Can you work these out from the drawing? Everything is in mm from the part's minimum corner. A direction names the side the tool comes from. Coordinates: 2 decimals unless noted, no trailing zeros. Order: outer loops, then holes, each group sorted by start corner. A loop starts at its lowest first (then second) coordinate and runs counter-clockwise, first axis right, second up. Notation, with made-up numbers: (19, 48) -> (62, 48) arc R15 ccw to (62, 61) -> close; hole circle Ø8 at (43.5, 42.5). An arc over 180 degrees is marked (long way). Answer in a Markdown table with one row per item.
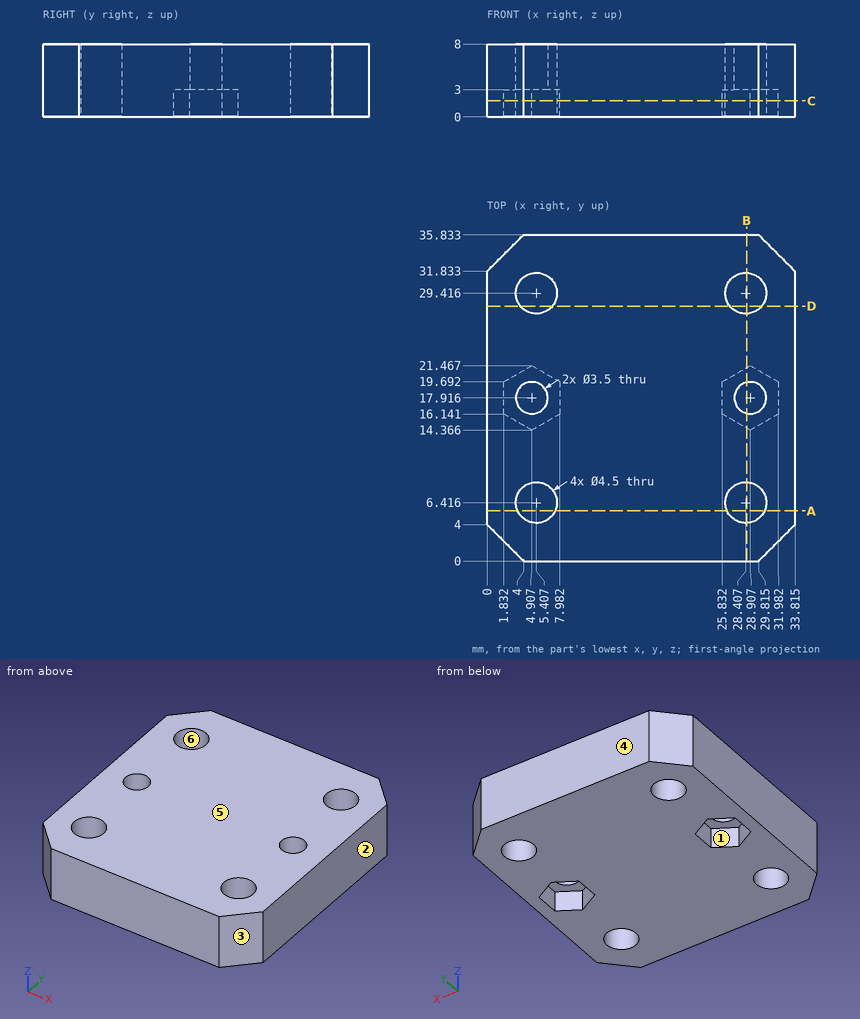
(1) Suppose I cut it at D-D (y = 28). Please give me the cut outline in (x, z) (1 decimal).
Response values:
| item | result |
|---|---|
| outline | (0, 0) -> (3.7, 0) -> (3.7, 8) -> (0, 8) -> close; (7.2, 0) -> (26.7, 0) -> (26.7, 8) -> (7.2, 8) -> close; (30.2, 0) -> (33.8, 0) -> (33.8, 8) -> (30.2, 8) -> close |
(2) Suppose I cut it at C-C (z = 1.75). Count the separate pieces of the cut face and the enclosed holes in it, and give its area (3 significant figures).
Response values:
| item | result |
|---|---|
| separate pieces | 1 |
| enclosed holes | 6 |
| area | 1,050 mm2 |
(3) Suppose I cut it at A-A (y = 5.5). Please give me the cut outline in (x, z) (1 decimal), and give its area (3 significant figures).
Response values:
| item | result |
|---|---|
| outline | (0, 0) -> (3.4, 0) -> (3.4, 8) -> (0, 8) -> close; (7.5, 0) -> (26.4, 0) -> (26.4, 8) -> (7.5, 8) -> close; (30.5, 0) -> (33.8, 0) -> (33.8, 8) -> (30.5, 8) -> close |
| area | 205 mm2 |
(4) Will this pin go through, and if not, where does the flat tip stop? pin 1 Ø4 at (x, y) = (4.91, 17.92) entering from -Z.
Response values:
| item | result |
|---|---|
| pin 1 | z = 3 |
(5) On a 3-axis mill with a long thin cutter (end or side, diameter ignored), from which of +Z, -Z, +X, -X, +Y, -Y can I reach the whole of each face in a straight line? I mean the marked faces 1 and 2. Say none if no direction works.
Response values:
| item | result |
|---|---|
| face 1 | -Z |
| face 2 | +Z, -Z, +X, +Y, -Y |
(6) I need wall thicknesses on line 1 (X direction, y = 18.5, z = 5.5) (1 decimal); line 2 (X direction, y = 29, z = 5.25) (1 decimal); line 3 (X direction, y = 34, z = 7) (1 decimal). Which ranges of each line are inside material? Lowest first, please. Write a range as [from, to].
Response values:
| item | result |
|---|---|
| line 1 | [0, 3.3], [6.6, 27.3], [30.6, 33.8] |
| line 2 | [0, 3.2], [7.6, 26.2], [30.6, 33.8] |
| line 3 | [2.2, 31.6] |
(7) Suppose I cut it at B-B (x = 28.5). Please give me the cut outline in (y, z) (1 decimal).
Response values:
| item | result |
|---|---|
| outline | (0, 0) -> (4.2, 0) -> (4.2, 8) -> (0, 8) -> close; (8.7, 0) -> (14.6, 0) -> (14.6, 3) -> (16.2, 3) -> (16.2, 8) -> (8.7, 8) -> close; (19.6, 3) -> (21.2, 3) -> (21.2, 0) -> (27.2, 0) -> (27.2, 8) -> (19.6, 8) -> close; (31.7, 0) -> (35.8, 0) -> (35.8, 8) -> (31.7, 8) -> close |
(8) We'd pull the mould along Y, two halves only. Please class the marked faces 3, 4, 5 and 6: +Y half, -Y half, draft (parallel to the pull), parting line (faces both ways), or undercut.
Response values:
| item | result |
|---|---|
| face 3 | -Y half |
| face 4 | +Y half |
| face 5 | draft |
| face 6 | undercut |
